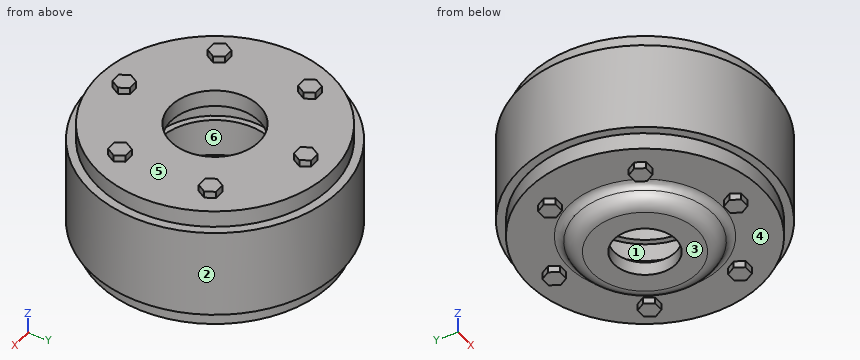
```python
from build123d import *

# Parameters (mm, degrees)
SKETCH_2_R                    = 37.5
SKETCH_2_R_2                  = 34.5
EXTRUDE_1_DEPTH               = 3
SKETCH_3_R                    = 70
SKETCH_3_R_2                  = 26.5
EXTRUDE_2_DEPTH               = 10
EXTRUDE_3_DEPTH               = 4
PATTERN_CIRCULAR_1_COUNT      = 6
PATTERN_LINEAR_1_COUNT        = 2
PATTERN_LINEAR_1_PITCH        = 77
PATTERN_LINEAR_1_COPY_1_DEPTH = 4
PATTERN_LINEAR_1_COPY_2_DEPTH = 4
PATTERN_LINEAR_1_COPY_3_DEPTH = 4
PATTERN_LINEAR_1_COPY_4_DEPTH = 4
PATTERN_LINEAR_1_COPY_5_DEPTH = 4


with BuildPart() as part:
    # 草图1 → 旋转1 (revolve)
    with BuildSketch(Plane(origin=(0, 0, 0), x_dir=(1, 0, 0), z_dir=(0, 1, 0))):
        Polygon((37.5, 26.5), (37.5, 11.25), (34, 11.25), (34, -11.25), (37.5, -11.25), (37.5, -26.5), (75, -26.5), (75, 26.5), align=None)
    revolve(axis=Axis((0, 0, 1000), (0, 0, -1)))

    # 草图2 → 凸台-拉伸1 (add)
    with BuildSketch(Plane.XY.offset(26.5)):
        Circle(SKETCH_2_R)
        Circle(SKETCH_2_R_2, mode=Mode.SUBTRACT)
    extrude(amount=-EXTRUDE_1_DEPTH)

    # 草图3 → 凸台-拉伸2 (add)
    with BuildSketch(Plane.XY.offset(26.5)):
        Circle(SKETCH_3_R)
        Circle(SKETCH_3_R_2, mode=Mode.SUBTRACT)
    extrude(amount=EXTRUDE_2_DEPTH)

    # 草图4 → 旋转2 (revolve)
    with BuildSketch(Plane(origin=(0, 0, 0), x_dir=(0, 0, -1), z_dir=(1, 0, 0)), mode=Mode.PRIVATE) as revolve_2_sk:
        with BuildLine():
            Line((26.5, 37.5), (26.5, 70))
            Line((26.5, 70), (36.5, 70))
            Line((36.5, 70), (36.5, 45.642135624))
            ThreePointArc((36.5, 45.642135624), (37.417517095, 42.755384278), (39.833333333, 40.928090416))
            ThreePointArc((39.833333333, 40.928090416), (44.664965809, 37.273502692), (46.5, 31.5))
            Line((46.5, 31.5), (46.5, 18.5))
            Line((46.5, 18.5), (38.5, 18.5))
            Line((38.5, 18.5), (38.5, 24.5))
            ThreePointArc((38.5, 24.5), (35.571067812, 31.571067812), (28.5, 34.5))
            Line((28.5, 34.5), (24.5, 34.5))
            Line((24.5, 34.5), (24.5, 37.5))
            Line((24.5, 37.5), (26.5, 37.5))
        make_face()
    revolve(revolve_2_sk.sketch.rotate(Axis((0, 0, 1000), (0, 0, -1)), 90), axis=Axis((0, 0, 1000), (0, 0, -1)))

    # 草图5 → 凸台-拉伸3 (add)
    with BuildSketch(Plane.XY.offset(36.5)):
        Polygon((3, 48.803847577), (6, 54), (3, 59.196152423), (-3, 59.196152423), (-6, 54), (-3, 48.803847577), align=None)
    extrude_3 = extrude(amount=EXTRUDE_3_DEPTH)

    # 阵列(圆周)1: 凸台-拉伸3 ×6 about axis
    pattern_circular_1_axis = Axis((0, 0, 0), (0, 0, 1))
    for i in range(1, PATTERN_CIRCULAR_1_COUNT):
        add(extrude_3.rotate(pattern_circular_1_axis, i * 360 / PATTERN_CIRCULAR_1_COUNT))

    # 阵列(线性)1: 凸台-拉伸3 ×2
    with Locations(*[(0, 0, -i * PATTERN_LINEAR_1_PITCH) for i in range(1, PATTERN_LINEAR_1_COUNT)]):
        add(extrude_3)

    # 阵列(线性)1 copy 1 sketch → 阵列(线性)1 copy 1 (add)
    with BuildSketch(Plane(origin=(0, 0, -40.5), x_dir=(0.5000000000000001, 0.8660254037844386, 0), z_dir=(0, 0, 1))):
        Polygon((3, 48.803847577), (6, 54), (3, 59.196152423), (-3, 59.196152423), (-6, 54), (-3, 48.803847577), align=None)
    extrude(amount=PATTERN_LINEAR_1_COPY_1_DEPTH)

    # 阵列(线性)1 copy 2 sketch → 阵列(线性)1 copy 2 (add)
    with BuildSketch(Plane(origin=(0, 0, -40.5), x_dir=(-0.4999999999999998, 0.8660254037844387, 0), z_dir=(0, 0, 1))):
        Polygon((3, 48.803847577), (6, 54), (3, 59.196152423), (-3, 59.196152423), (-6, 54), (-3, 48.803847577), align=None)
    extrude(amount=PATTERN_LINEAR_1_COPY_2_DEPTH)

    # 阵列(线性)1 copy 3 sketch → 阵列(线性)1 copy 3 (add)
    with BuildSketch(Plane(origin=(0, 0, -40.5), x_dir=(-1, 0, 0), z_dir=(0, 0, 1))):
        Polygon((3, 48.803847577), (6, 54), (3, 59.196152423), (-3, 59.196152423), (-6, 54), (-3, 48.803847577), align=None)
    extrude(amount=PATTERN_LINEAR_1_COPY_3_DEPTH)

    # 阵列(线性)1 copy 4 sketch → 阵列(线性)1 copy 4 (add)
    with BuildSketch(Plane(origin=(0, 0, -40.5), x_dir=(-0.5000000000000004, -0.8660254037844384, 0), z_dir=(0, 0, 1))):
        Polygon((3, 48.803847577), (6, 54), (3, 59.196152423), (-3, 59.196152423), (-6, 54), (-3, 48.803847577), align=None)
    extrude(amount=PATTERN_LINEAR_1_COPY_4_DEPTH)

    # 阵列(线性)1 copy 5 sketch → 阵列(线性)1 copy 5 (add)
    with BuildSketch(Plane(origin=(0, 0, -40.5), x_dir=(0.5000000000000001, -0.8660254037844386, 0), z_dir=(0, 0, 1))):
        Polygon((3, 48.803847577), (6, 54), (3, 59.196152423), (-3, 59.196152423), (-6, 54), (-3, 48.803847577), align=None)
    extrude(amount=PATTERN_LINEAR_1_COPY_5_DEPTH)


solid = part.part
```
The listing builds one solid part. Answer for the finished solid, in the listing's coordinates (mm). Face numbers are marked on the shaded views. A direction names the side the tool comes from. Give positions to 0.01 mm unless a question says otherwise; leave off trailing zeros. Order: outer loops, then holes, each group sorted by start corner. A loop starts at its lowest first (then second) coordinate and runs counter-clockwise, first axis right, second up.
1) Consider line 1 along Y through (x, z) = (0, 0.25); line 2 along Y through (x, z) = (0, -25). Determine where each line is inside the solid, lowest interval first.
Reported:
line 1: y = -75 to -34, 34 to 75
line 2: y = -75 to -34.5, 34.5 to 75
2) Determine the mould class of the marked faces 1, 2 and 3 for opening direction X: pulls with the +X half, pulls with the -X half, needs draft (parallel to the pull), parting line crosses it, or undercut.
Reported:
face 1: undercut
face 2: parting line crosses it
face 3: needs draft
3) Find section A-A on z = 17. Write down the section's boundary in (x, y), then the cut area to 3 significant figures.
Reported:
outline: circle Ø150 at (0, 0); hole circle Ø75 at (0, 0)
area: 13,300 mm2
4) For the marked faces 4, 5 and 6, determine the directions among +Z, -Z, +X, -X, +Y, -Y from which every point of the face is accessible in a straight line to the end or side of a thin tool.
Reported:
face 4: -Z
face 5: +Z
face 6: none
5) Given P1, Ø6, axis at x = 40.5, y = 39.5, coming from the -Z side; P2, Ø3, axis at x = -46.5, y = 27, coming from the -Z side; P3, Ø2, axis at x = 46.5, z = -38.5, coming from the +Y side, each flat-ended and moving along its own axis, determine where each tip first touches the part or whether it passes through.
Reported:
P1: stops at z = -36.5
P2: stops at z = -40.5
P3: stops at y = 32.2
6) Find section B-B on y = -63. Write down the section's boundary in (x, z), then the cut area to 3 significant figures.
Reported:
outline: (-40.69, -26.5) - (-30.51, -26.5) - (-30.51, -36.5) - (30.51, -36.5) - (30.51, -26.5) - (40.69, -26.5) - (40.69, 26.5) - (30.51, 26.5) - (30.51, 36.5) - (-30.51, 36.5) - (-30.51, 26.5) - (-40.69, 26.5) - close
area: 5,530 mm2
